```python
from build123d import *

# Parameters (mm, degrees)
F2_R = 0.254


with BuildPart() as f1:
    # F0 (on Top) → F1 (revolve)
    with BuildSketch(Plane.XY):
        Polygon((-12.3952, 0), (-3.2385, 0), (-3.2385, 1.905), (-7.10248, 6.35), (-10.203748, 6.35), (-12.3952, 4.445), align=None)
    revolve(axis=Axis((0, 4.669294, 0), (0, 1, 0)))

    # F2
    f2_edges = [f1.edges().sort_by_distance(p)[0] for p in [
        (12.3952, 4.445, 0),
        (10.203748, 6.35, 0),
    ]]
    fillet(f2_edges, radius=F2_R)


solid = f1.part
```
Design review of the part built by this model. Coordinates are the model's own, in mm. Give positions to 0.01 mm unless a question says otherwise; leave off trailing zeros. Write item = value, one per line. Start each with the question number.
(1) For pin 1 (3 mm diameter, centred on x = 4.5, y = 2, fed in from -Z), flat-tipped, find the tip position at first contact; note if it passes through.
(2) Mouldability with a two-part tool opening along X and no side actions: class faces 1 (the face through (0.8, 2.2, -3.4)), 2 (the face through (-7, 6.35, -2)), 3 (the face through (-11.45, 2.13, -4.75)) as +X half, -X half, draft (parallel to the pull), parting line (faces both ways), or undercut.
(3) To check wall thickness, follow line 1 along Z through (x, y) = (0, 0.65); line 2 along X through (y, z) = (5.25, -2.5); line 3 along Z through (x, y) = (3.25, 3.5). State the ranges of each line that lie inside material, in increasing order.
Numbers:
q1.pin_1 = -12.03
q2.face_1 = undercut
q2.face_2 = draft
q2.face_3 = parting line
q3.line_1 = -12.4 to -3.24, 3.24 to 12.4
q3.line_2 = -11.19 to -5.61, 5.61 to 11.19
q3.line_3 = -11.96 to -3.29, 3.29 to 11.96
